Design review of the part shown in the three views and the two pictorial views. Dimensions are in mm from the part's minimum x, y and z. A direction names the side the tool comes from. Round coordinates to 2 decimals unless told otherwise and drop trailing zeros. Loops run counter-clockwise (first coordinate to the right, second up) from the corner with the lowest first, then second, coordinate; pieces in that order, holes last. Notation, with made-up numbers: (25.25, -31) -> (74.25, -31) arc R21 cw to (74.25, -21) -> close; hole circle Ø9 at (87, -6). An arc over 180 degrees is marked (long way). One line per question, with ' | ' between items. Start each with the question number.
1. Consider section B-B (y = 9). Write out the cut boundary in (x, z), and give its area (3 significant figures).
2. Consider section D-D (y = 1). Write out the cut boundary in (x, z).
3. For pin 1 Ø2 at (x, z) = (6, 14) entering from -Y; pin 2 Ø1.5 at (x, y) = (29.5, 8) entering from -Z; pin 3 Ø2 at (y, z) = (2.5, 4) entering from -X; pin 4 Ø3 at (x, z) = (20, 14) entering from -Y, all flat-tipped, find the tip position at first contact; note any pin that passes through.
4. Consider section C-C (x = 20). Write out the cut boundary in (y, z), and give its area (3 significant figures).
5. Consider section A-A (z = 12.5). Write out the cut boundary in (x, y).
6. Wall thickness on line 1 along Z through (x, y) = (20, 8.9); line 2 along Z through (x, y) = (30.5, 7.75); line 3 along X through (y, z) = (4, 7.5): over which ranges is each line inside the solid? List them lowest first.
7. Draft analysis for pull direction X (two halves, no side actions). For the marked faces 3, 4 and 5, state which applies: pulls with the +X half, pulls with the -X half, needs draft (parallel to the pull), parting line crosses it, or undercut.
8. For the marked faces 1 and 2, list the 3-axis set-ups (+Z, -Z, +X, -X, +Y, -Y) from which the entire face can be reached by the end or side of a thin tool; tool diameter is ignored.
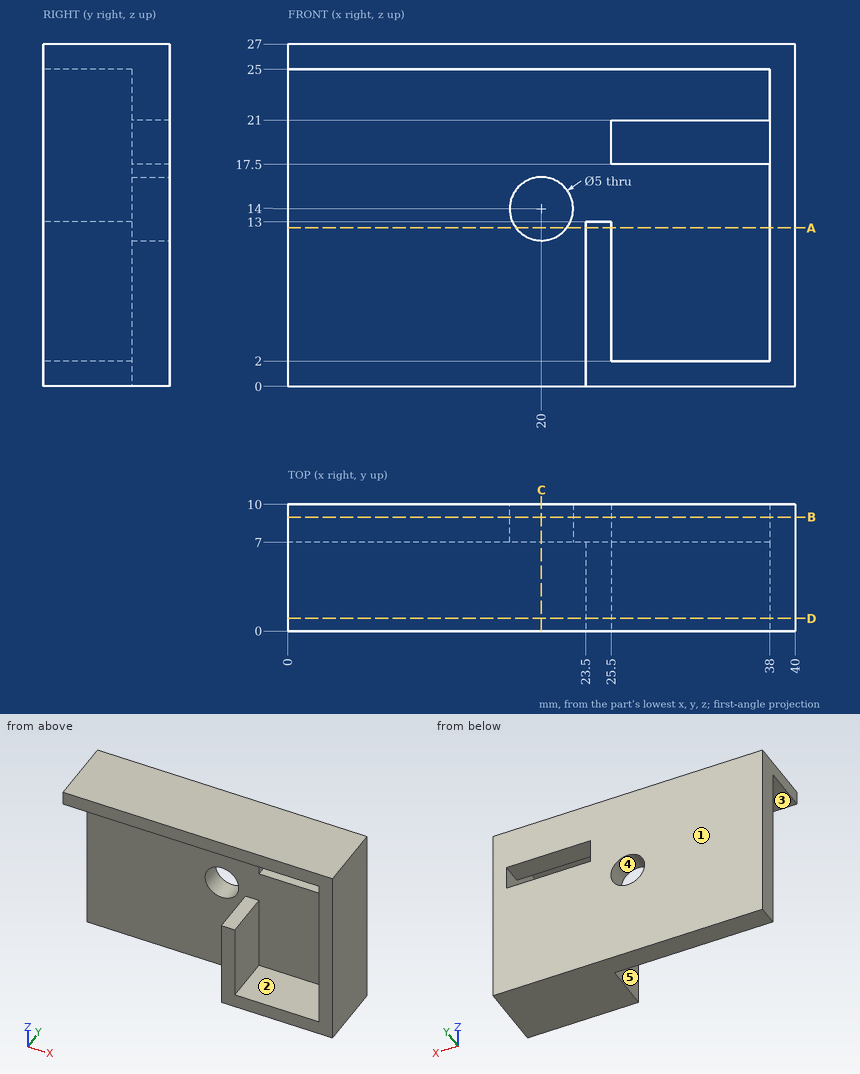
Answer block:
1) outline: (0, 0) -> (40, 0) -> (40, 27) -> (0, 27) -> close; hole circle Ø5 at (20, 14); hole (25.5, 17.5) -> (38, 17.5) -> (38, 21) -> (25.5, 21) -> close | area: 1,020 mm2
2) outline: (0, 25) -> (38, 25) -> (38, 2) -> (25.5, 2) -> (25.5, 13) -> (23.5, 13) -> (23.5, 0) -> (40, 0) -> (40, 27) -> (0, 27) -> close
3) pin 1: stops at y = 7 | pin 2: stops at z = 0 | pin 3: stops at x = 23.5 | pin 4: passes through
4) outline: (0, 25) -> (7, 25) -> (7, 16.5) -> (10, 16.5) -> (10, 27) -> (0, 27) -> close; (7, 0) -> (10, 0) -> (10, 11.5) -> (7, 11.5) -> close | area: 80.0 mm2
5) outline: (0, 7) -> (18, 7) -> (18, 10) -> (0, 10) -> close; (22, 7) -> (23.5, 7) -> (23.5, 0) -> (25.5, 0) -> (25.5, 7) -> (38, 7) -> (38, 0) -> (40, 0) -> (40, 10) -> (22, 10) -> close
6) line 1: z = 0 to 11.5, 16.5 to 27 | line 2: z = 0 to 17.5, 21 to 27 | line 3: x = 23.5 to 25.5, 38 to 40
7) face 3: needs draft | face 4: undercut | face 5: pulls with the -X half
8) face 1: +Z, -Z, +X, -X, +Y | face 2: -Y
